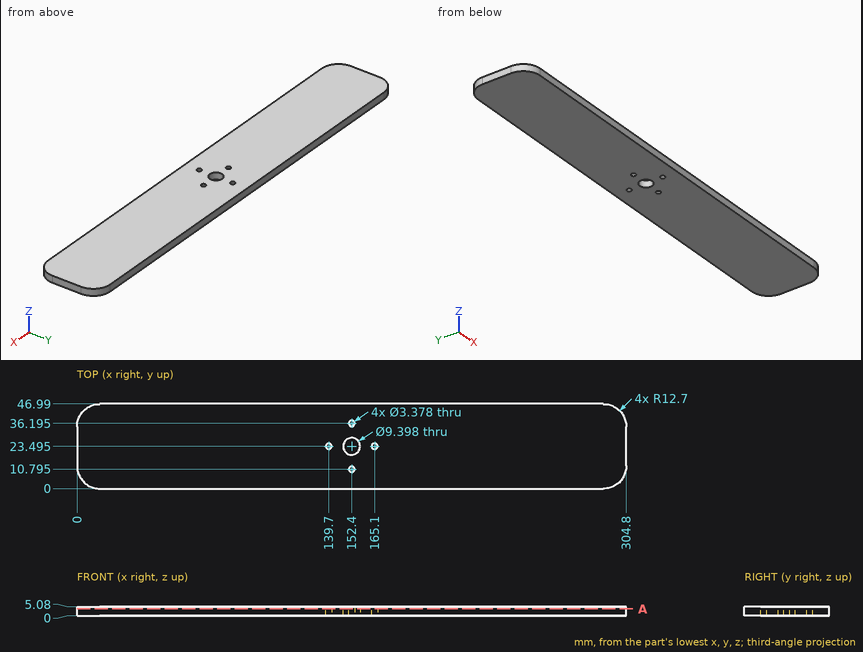
Drawing for the job (mm, zero at the part's lowest x, y, z). Round coordinates to 2 decimals unless told otherwise and drop trailing zeros. Write each loop counter-clockwise with the first axis right and the second up, starting at its lowest first coordinate (ties: lowest second). Pieces come first, ordered by that corner, then holes. Notation, with made-up numbers: (7, 76.5) - (35, 76.5) arc R36 cw to (35, 113.5) - close; hole circle Ø8 at (34.25, 10.25). An arc over 180 degrees is marked (long way). Write item = value, one per line. Start each with the question number.
Q1. Band-saw the part on A-A (z = 3.85). Give the cut face in (x, y) (1 decimal).
Q2. Probe L1, parallel to Y at x = 165, z = 1.35; L2, parallel to X at y = 36, z = 3.7; L3, parallel to X at y = 37.5, z = 3.3. List the from-to ranges inside material, lowest first. Write a range as from..to.
Q3. Drop a flat-ended pin along its axis: pin 1 (4.5 mm diameter, centred on x = 165.1, y = 23.495, fed in from +Z). Give the stop position or say it passes through.
Answers below:
q1.outline = (0, 12.7) arc R12.7 ccw to (12.7, 0) - (292.1, 0) arc R12.7 ccw to (304.8, 12.7) - (304.8, 34.3) arc R12.7 ccw to (292.1, 47) - (12.7, 47) arc R12.7 ccw to (0, 34.3) - close; hole circle Ø3.4 at (139.7, 23.5); hole circle Ø9.4 at (152.4, 23.5); hole circle Ø3.4 at (152.4, 10.8); hole circle Ø3.4 at (152.4, 36.2); hole circle Ø3.4 at (165.1, 23.5)
q2.L1 = 0..21.81, 25.18..46.99
q2.L2 = 0.12..150.72, 154.08..304.68
q2.L3 = 0.41..151.33, 153.47..304.39
q3.pin_1 = 5.08
